Check sheet for the modelled part. Datum: model origin and axes. Units: mm. Face numbers are marked on the shaded views. Round coordinates to 2 decimals unless told otherwise and drop trailing zeros. Write each loop counter-clockwise with the first axis right and the second up, starting at its lowest first coordinate (ties: lowest second). Pieces come first, ordered by that corner, then holes. Notation, with made-up numbers: (35, -1.5) -> (94, -1.5) arc R25 cw to (94, 32.5) -> close; hole circle Ø10 at (-13.5, 5). An arc over 180 degrees is marked (long way). Write item = value, one per line.
Solid Edge part; units mm, degrees
sketch "Sketch1" plane through (0, 0, 0) normal (0, 0, 1) x (1, 0, 0)
  spline S0 degree 3 poles (-0.2928, 1.9785) (-0.306, 2.1503) (-0.3512, 2.501) (-0.5844, 2.7739) (-0.7056, 2.9158) knots 0 0 0 0 0.479886 1 1 1 1
  arc A0 (-0.7056, 2.9158) -> (-1.143, 2.7737) centre (0, 0) ccw
  spline S1 degree 3 poles (-0.926, 1.7727) (-1.0163, 1.9195) (-1.1859, 2.2298) (-1.1577, 2.5876) (-1.143, 2.7737) knots 0 0 0 0 0.479886 1 1 1 1
  arc A1 (-0.926, 1.7727) -> (-0.2928, 1.9785) centre (0, 0) cw
extrude "Protrusion1" add sketch "Sketch1" along normal blind 4
sketch "Sketch2" plane through (0, 0, 0) normal (0, 0, 1) x (1, 0, 0)
  circle A0 centre (0, 0) radius 1
  circle A1 centre (0, 0) radius 2
extrude "Rad" add sketch "Sketch2" along normal blind 4
pattern_circular "Pattern1" count 10 over 360 about axis through (0, 0, 0) along (0, 0, 1) of "Protrusion1"
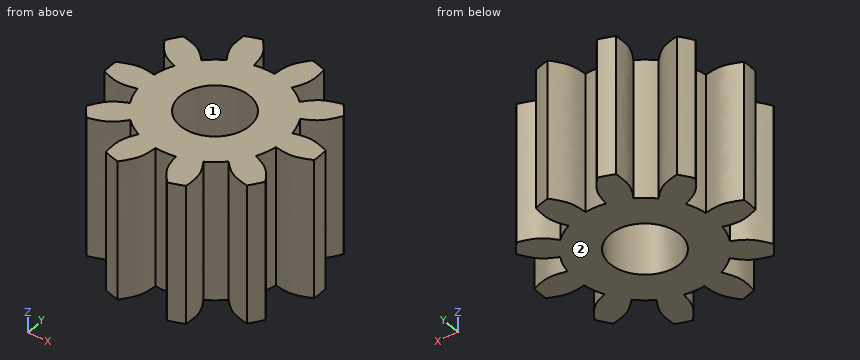
(1) Material ranges on L1, parallel to Y at x = 0, z = 2.4; L2, parallel to Y at x = 2, z = 3.4; L3, parallel to Y at x = 0.75, z = 1.85, recorded low to high. Write a range as [from, to].
Worked answers:
L1 = [-2, -1], [1, 2]
L2 = [-1.87, -0.99], [-0.34, 0.34], [0.99, 1.87]
L3 = [-2.9, -0.66], [0.66, 2.9]
(2) Release check for a two-part mould opening along Y. For the marked faces 1 and 2 record: pulls with the +Y half, pulls with the -Y half, needs draft (parallel to the pull), parting line crosses it, or undercut.
Worked answers:
face_1 = undercut
face_2 = needs draft
(3) Go/stop test with flat-tipped pins: P1, Ø2, axis at y = -1.5, z = 2.5, coming from the +X side; P2, Ø1, axis at x = 0, z = 1.5, coming from the -Y side. Record where each tip stops, or that it passes through.
Worked answers:
P1 = 2.56
P2 = -2.66
(4) Sectioned sample at A-A on x = 0. Enter the section's corners in (y, z).
Worked answers:
outline = (-2, 0) -> (-1, 0) -> (-1, 4) -> (-2, 4) -> close; (1, 0) -> (2, 0) -> (2, 4) -> (1, 4) -> close
(5) Sectioned sample at B-B on y = 0. Enter the section's corners in (x, z), then the cut area to 3 significant figures.
Worked answers:
outline = (-3, 0) -> (-1, 0) -> (-1, 4) -> (-3, 4) -> close; (1, 0) -> (3, 0) -> (3, 4) -> (1, 4) -> close
area = 16.0 mm²
